from build123d import *

# Parameters (mm, degrees)
SKETCH2_W           = 38.1
SKETCH2_H           = 76.2
BOSS_EXTRUDE1_DEPTH = 12.7
SKETCH5_W           = 38.1
SKETCH5_H           = 18.614666354
BOSS_EXTRUDE5_DEPTH = 2.54
SKETCH4_R           = 1.905
BOSS_EXTRUDE6_DEPTH = 10.16
SKETCH7_W           = 38.1
SKETCH7_H           = 18.614666354
BOSS_EXTRUDE7_DEPTH = 3.81


with BuildPart() as part:
    # Sketch2 → Boss-Extrude1 (new body)
    with BuildSketch(Plane(origin=(0, 0, 0), x_dir=(1, 0, 0), z_dir=(0, 1, 0))):
        with Locations((19.05, 38.1)):
            Rectangle(SKETCH2_W, SKETCH2_H)
    extrude(amount=BOSS_EXTRUDE1_DEPTH)

    # Sketch5 → Boss-Extrude5 (add)
    with BuildSketch(Plane(origin=(0, 12.7, 0), x_dir=(1, 0, 0), z_dir=(0, 1, 0))):
        with Locations((19.05, 9.307333177)):
            Rectangle(SKETCH5_W, SKETCH5_H)
    extrude(amount=BOSS_EXTRUDE5_DEPTH)

    # Sketch4 → Boss-Extrude6 (add)
    with BuildSketch(Plane(origin=(38.1, 0, 0), x_dir=(0, 0, -1), z_dir=(1, 0, 0))):
        with Locations(Location((25.4, 6.35, 0), (0, 0, 180))):
            Circle(SKETCH4_R)
    extrude(amount=BOSS_EXTRUDE6_DEPTH)

    # Sketch7 → Boss-Extrude7 (add)
    with BuildSketch(Plane(origin=(0, 15.24, 0), x_dir=(1, 0, 0), z_dir=(0, 1, 0))):
        with Locations((19.05, 9.307333177)):
            Rectangle(SKETCH7_W, SKETCH7_H)
    extrude(amount=BOSS_EXTRUDE7_DEPTH)


solid = part.part
Geometry: final body of the model. Coordinates: model frame, mm. A direction names the side the tool comes from. Give positions to 0.01 mm unless a question says otherwise; leave off trailing zeros. Order: outer loops, then holes, each group sorted by start corner. A loop starts at its lowest first (then second) coordinate and runs counter-clockwise, first axis right, second up. Notation, with made-up numbers: (-20, 69) -> (21, 69) arc R30 cw to (21, 98) -> close; hole circle Ø4 at (73, 46.5). An arc over 180 degrees is marked (long way). Put each result on its own line as item: value.
Q1. Section A-A, the plane x = 8. Return loops of the section in (y, z).
Here are the results:
outline: (0, -76.2) -> (12.7, -76.2) -> (12.7, -18.61) -> (19.05, -18.61) -> (19.05, 0) -> (0, 0) -> close
Q2. Pin query (flat end, axial travel): pin 1 (12 mm diameter, centred on x = 11, z = -26, fed in from +Y); pin 2 (3 mm diameter, centred on x = 13, y = 15, fed in from -Z). Return the tip coordinate at first contact, or that it passes through.
Here are the results:
pin 1: stops at y = 12.7
pin 2: stops at z = -18.61
Q3. Section B-B, the plane y = 6.35. Return loops of the section in (x, z) (3 decimals), then the cut area to 3 significant figures.
Here are the results:
outline: (0, -76.2) -> (38.1, -76.2) -> (38.1, -27.305) -> (48.26, -27.305) -> (48.26, -23.495) -> (38.1, -23.495) -> (38.1, 0) -> (0, 0) -> close
area: 2,940 mm^2
Q4. Material intervals for L1, parallel to Y at x = 12, z = -65; L2, parallel to X at y = 1.75, z = -72; L3, parallel to Z at x = 10, y = 17.75, sorted ascending.
Here are the results:
L1: y = 0 to 12.7
L2: x = 0 to 38.1
L3: z = -18.61 to 0
Q5. Section C-C, the plane z = -25.4. Return loops of the section in (x, y) (3 decimals), then the cut area to 3 significant figures.
Here are the results:
outline: (0, 0) -> (38.1, 0) -> (38.1, 4.445) -> (48.26, 4.445) -> (48.26, 8.255) -> (38.1, 8.255) -> (38.1, 12.7) -> (0, 12.7) -> close
area: 523 mm^2
Q6. Section D-D, the plane z = -8.5. Return loops of the section in (x, y).
Here are the results:
outline: (0, 0) -> (38.1, 0) -> (38.1, 19.05) -> (0, 19.05) -> close
Q7. Reachability of faces 1 (the face through (0, 7, -38)), 2 (the face through (43.11, 7.51, -26.91)), 3 (the face through (19, 12.7, -48)) from +Z, -Z, +X, -X, +Y, -Y: full face, straight path, thin tool, end or side. Return the list, or none.
Here are the results:
face 1: +Z, -Z, -X, +Y, -Y
face 2: +X
face 3: -Z, +X, -X, +Y
